Input: part model. Units: mm. Frame: model coordinates. A direction names the side the tool comes from. Give positions to 0.01 mm unless a question says otherwise; leave off trailing zeros. Loops run counter-clockwise (first coordinate to the right, second up) from the corner with the lowest first, then second, coordinate; pieces in that order, holes last. Notation, with made-up numbers: (-26, 12) - (-7, 12) arc R12 ccw to (-7, 30) - close; hole circle Ø10 at (36.25, 26.5). An arc over 180 degrees is marked (long way). Answer as a JSON object with one key per item and string values.
from build123d import *

# Parameters (mm, degrees)
SKETCH1_R           = 10
SKETCH1_R_2         = 2.5
SKETCH1_R_3         = 1.5
BOSS_EXTRUDE1_DEPTH = 1.8
SKETCH2_R           = 3.5
SKETCH2_R_2         = 2.5
BOSS_EXTRUDE2_DEPTH = 2.7
SKETCH3_R           = 2.5
BOSS_EXTRUDE3_DEPTH = 1


with BuildPart() as part:
    # Sketch1 → Boss-Extrude1 (new body)
    with BuildSketch(Plane(origin=(0, 0, 0), x_dir=(1, 0, 0), z_dir=(0, 1, 0))):
        Circle(SKETCH1_R)
        Circle(SKETCH1_R_2, mode=Mode.SUBTRACT)
        with Locations((0, 7)):
            Circle(SKETCH1_R_3, mode=Mode.SUBTRACT)
        with Locations((7, 0)):
            Circle(SKETCH1_R_3, mode=Mode.SUBTRACT)
        with Locations((0, -7)):
            Circle(SKETCH1_R_3, mode=Mode.SUBTRACT)
        with Locations((-7, 0)):
            Circle(SKETCH1_R_3, mode=Mode.SUBTRACT)
    extrude(amount=BOSS_EXTRUDE1_DEPTH)

    # Sketch2 → Boss-Extrude2 (add)
    with BuildSketch(Plane(origin=(0, 1.8, 0), x_dir=(1, 0, 0), z_dir=(0, 1, 0))):
        Circle(SKETCH2_R)
        Circle(SKETCH2_R_2, mode=Mode.SUBTRACT)
    extrude(amount=BOSS_EXTRUDE2_DEPTH)

    # Sketch3 → Boss-Extrude3 (add)
    with BuildSketch(Plane(origin=(0, 0, 0), x_dir=(-1, 0, 0), z_dir=(0, -1, 0))):
        Circle(SKETCH3_R)
    extrude(amount=-BOSS_EXTRUDE3_DEPTH)


solid = part.part
Item 1: Cut plane A-A (x = 0). Return loops of the section in (y, z).
Geometry check:
{"outline": "(0, -10) - (1.8, -10) - (1.8, -8.5) - (0, -8.5) - close; (0, -5.5) - (1.8, -5.5) - (1.8, -3.5) - (4.5, -3.5) - (4.5, -2.5) - (1, -2.5) - (1, 2.5) - (4.5, 2.5) - (4.5, 3.5) - (1.8, 3.5) - (1.8, 5.5) - (0, 5.5) - close; (0, 8.5) - (1.8, 8.5) - (1.8, 10) - (0, 10) - close"}
Item 2: Cut plane D-D (y = 0.65). Return loops of the section in (x, z), then the cut area to 3 significant figures.
Geometry check:
{"outline": "circle Ø20 at (0, 0); hole circle Ø3 at (-7, 0); hole circle Ø3 at (0, -7); hole circle Ø3 at (0, 7); hole circle Ø3 at (7, 0)", "area": "286 mm2"}
Item 3: Access query for faces 4 (the face through (-0.54, 2.73, 2.44)), 5 (the face through (-2.17, 0.89, 9.76)). Directions: +Z, -Z, +X, -X, +Y, -Y. A direction counts if a zero-diameter tool reaches every point of the face in a straight line with its end or side. Return the directions, or none.
Geometry check:
{"face 4": "+Y", "face 5": "+Y, -Y"}
Item 4: Mould query, pull axis Z, two halves, no side actions, for faces 1 (the face through (3.233, 3.131, 1.341)), 2 (the face through (2, 4.5, 2)), 3 (the face through (-0.325, 0.887, -5.536)). Classes: released by +Z, released by -Z, zero draft, split by the parting line, or undercut.
Geometry check:
{"face 1": "split by the parting line", "face 2": "zero draft", "face 3": "undercut"}
Item 5: Contact query for flat-ended pins moving along their axis: P1, Ø2, axis at x = -6.5, y = 4, coming from the +Z side; P2, Ø4, axis at x = 7, z = 0, coming from the +Y side; P3, Ø1, axis at x = 2.5, y = 1.5, coming from the +Z side; P4, Ø2.5, axis at x = -0.5, z = 1, coming from the +Y side. Output: stop coordinate, or through.
Geometry check:
{"P1": "passes through", "P2": "stops at y = 1.8", "P3": "stops at z = 9.8", "P4": "stops at y = 1"}
Item 6: Material intervals for line 1 (Z direction, x = 0, y = 1.2); line 2 (X direction, y = 3.5, z = 0), sorted ascending. Write a range as [from, to].
Geometry check:
{"line 1": "z = [-10, -8.5], [-5.5, -2.5], [2.5, 5.5], [8.5, 10]", "line 2": "x = [-3.5, -2.5], [2.5, 3.5]"}
Item 7: Cut plane C-C (x = 7.5). Return loops of the section in (y, z), then the cut area to 3 significant figures.
Geometry check:
{"outline": "(0, -6.61) - (1.8, -6.61) - (1.8, -1.41) - (0, -1.41) - close; (0, 1.41) - (1.8, 1.41) - (1.8, 6.61) - (0, 6.61) - close", "area": "18.7 mm2"}
Item 8: Cut plane B-B (z = 7). Return loops of the section in (x, y), then the cut area to 3 significant figures.
Geometry check:
{"outline": "(-7.14, 0) - (-1.5, 0) - (-1.5, 1.8) - (-7.14, 1.8) - close; (1.5, 0) - (7.14, 0) - (7.14, 1.8) - (1.5, 1.8) - close", "area": "20.3 mm2"}
